Drawing for the job (mm, zero at the part's lowest x, y, z). A direction names the side the tool comes from. Round coordinates to 2 decimals unless told otherwise and drop trailing zeros. Loops run counter-clockwise (first coordinate to the right, second up) from the corner with the lowest first, then second, coordinate; pieces in that order, holes last. Notation, with made-up numbers: M -3.75,-28.75 L 47.25,-28.75 A18 ccw 47.25,-20.75 Z; hole C 14,66.5 d11. An arc over 180 degrees is marked long. Use a Markdown table: item, result. Add a question column.
Q1. Probe line 1 (X direction, y = 5.5, z = 40.5) (3 decimals); line 2 (Z direction, x = 33.5, y = 5.5); line 3 (Z direction, x = 29, y = 4.75). List the from-to ranges inside material, lowest first. Write a range as from..to.
Q2. Cut at B-B (z = 39.5). Give the cut face in (x, y) (3 decimals).
Q3. Cut at A-A (y = 4.5). Give the cut face in (x, z) (3 decimals), plus the area to 3 significant figures.
Q4. Tool access for the marked faces 1, 2 and 3: list every direction of +Z, -Z, +X, -X, +Y, -Y with a clear straight run to the whole face (end or side of a thin tool).
Q5. Pin check, flat tips, straight feed: pin 1 (1.9 mm diameter, centred on x = 6, y = 3.5, fed in from +Z); pin 2 (3 mm diameter, centred on y = 3.5, z = 41.5, fed in from +X) (3 decimals). Stop position of each tip, or through.
Q6. Cut at C-C (x = 4). Give the cut face in (y, z).
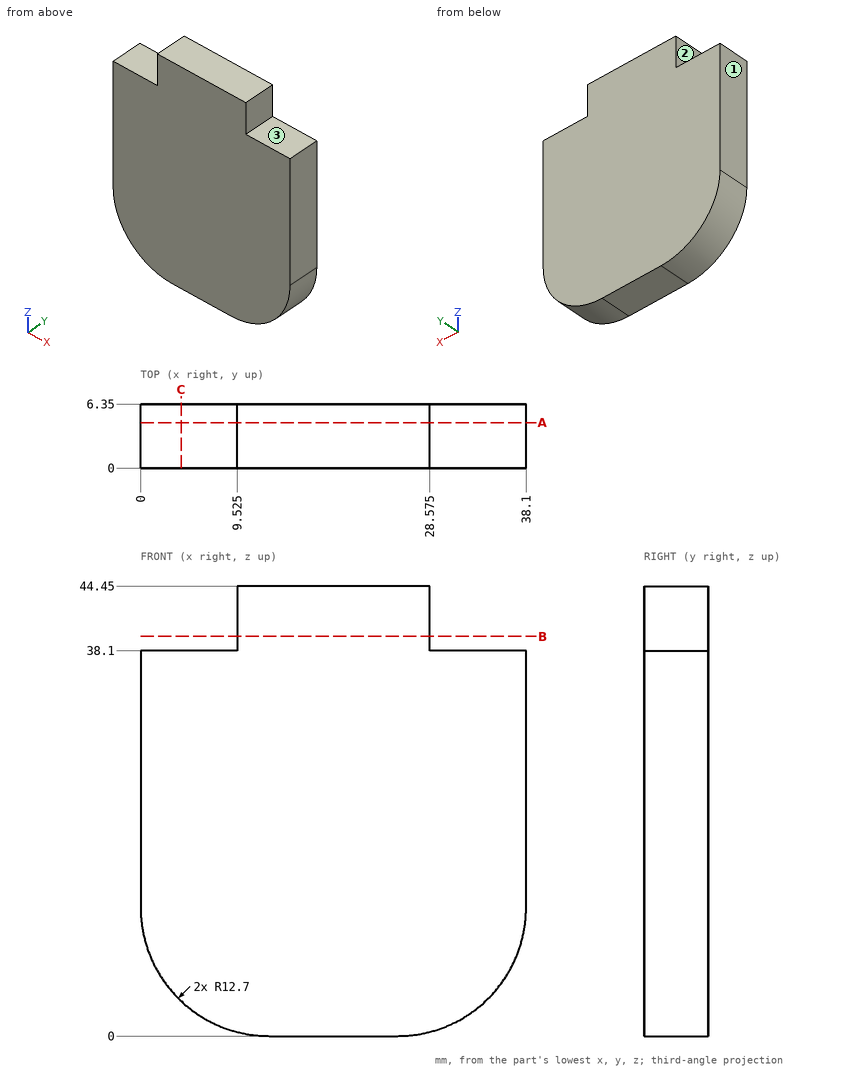
Checked values:
| question | item | result |
|---|---|---|
| 1 | line 1 | x = 9.525..28.575 |
| 1 | line 2 | z = 2.92..38.1 |
| 1 | line 3 | z = 0.52..38.1 |
| 2 | outline | M 9.525,0 L 28.575,0 L 28.575,6.35 L 9.525,6.35 Z |
| 3 | outline | M 0,12.7 A12.7 ccw 12.7,0 L 25.4,0 A12.7 ccw 38.1,12.7 L 38.1,38.1 L 28.575,38.1 L 28.575,44.45 L 9.525,44.45 L 9.525,38.1 L 0,38.1 Z |
| 3 | area | 1,500 mm^2 |
| 4 | face 1 | +Z, -Z, -X, +Y, -Y |
| 4 | face 2 | +Z, -X, +Y, -Y |
| 4 | face 3 | +Z, +X, +Y, -Y |
| 5 | pin 1 | stops at z = 38.1 |
| 5 | pin 2 | stops at x = 28.575 |
| 6 | outline | M 0,3.45 L 6.35,3.45 L 6.35,38.1 L 0,38.1 Z |
